Source: CAD feature listing. Evaluate the final solid. Frame: model axes, mm. Face numbers are marked on the shaded views. Give positions to 0.01 mm unless a question says otherwise; leave off trailing zeros. Write each loop counter-clockwise with the first axis right and the second up, starting at its lowest first coordinate (ties: lowest second). Pieces come first, ordered by that corner, then holes. Notation, with made-up numbers: (56.5, 31.5) -> (80.5, 31.5) arc R31 ccw to (80.5, 62.5) -> close; hole circle Ø7 at (82.25, -8). An arc over 180 degrees is marked (long way). Write item = value, one per line.
from build123d import *

# Parameters (mm, degrees)
BOSS_EXTRUDE1_DEPTH     = 432.4604
CUT_EXTRUDE1_DEPTH      = 18.43075
CUT_EXTRUDE1_DEPTH_BACK = 18.43075


with BuildPart() as part:
    # Sketch1 → Boss-Extrude1 (new body)
    with BuildSketch(Plane.XY):
        Polygon((-28.7655, -12.98575), (28.7655, -12.98575), (33.655, 17.43075), (38.1, 17.43075), (38.1, -17.43075), (-38.1, -17.43075), (-38.1, 17.43075), (-33.655, 17.43075), align=None)
    extrude(amount=BOSS_EXTRUDE1_DEPTH)

    # Sketch2 → Cut-Extrude1 (cut, two sides)
    with BuildSketch(Plane(origin=(0, 0, 0), x_dir=(1, 0, 0), z_dir=(0, 1, 0))) as cut_extrude1_sk:
        Polygon((-38.1, 0), (38.1, -129.9972), (38.1, 0), align=None)
        Polygon((-38.1, -432.4604), (38.1, -302.4632), (38.1, -432.4604), align=None)
    extrude(amount=CUT_EXTRUDE1_DEPTH, mode=Mode.SUBTRACT)
    extrude(cut_extrude1_sk.sketch, amount=-CUT_EXTRUDE1_DEPTH_BACK, mode=Mode.SUBTRACT)


solid = part.part
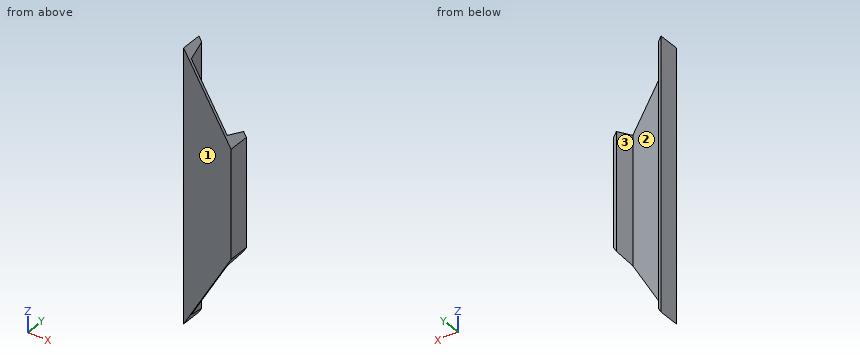
(1) First-contact query: pin 1 (6 mm diameter, centred on x = -21.5, z = 380, fed in from +Y); pin 2 (5 mm diameter, centred on y = 6, z = 65, fed in from +X). Flat tips, straight axial feed; report the tip coordinate or a pass-through.
Values follow:
pin_1 = -12.99
pin_2 = -31.42
(2) Section query B-B (z = 229.5). Return loops of the section in (x, y) (1 decimal), plus the area to 3 significant figures.
Values follow:
outline = (-38.1, -17.4) -> (38.1, -17.4) -> (38.1, 17.4) -> (33.7, 17.4) -> (28.8, -13) -> (-28.8, -13) -> (-33.7, 17.4) -> (-38.1, 17.4) -> close
area = 758 mm2
(3) Section query D-D (z = 382). Return loops of the section in (x, y) (1 decimal), plus the area to 3 significant figures.
Values follow:
outline = (-38.1, -17.4) -> (-8.5, -17.4) -> (-8.5, -13) -> (-28.8, -13) -> (-33.7, 17.4) -> (-38.1, 17.4) -> close
area = 341 mm2
(4) Section query A-A (y = 0). Return loops of the section in (x, z), plus the area to 3 significant figures.
Values follow:
outline = (-38.1, 0) -> (-30.85, 12.36) -> (-30.85, 420.1) -> (-38.1, 432.46) -> close; (30.85, 117.63) -> (38.1, 130) -> (38.1, 302.46) -> (30.85, 314.83) -> close
area = 4,380 mm2
(5) Section query C-C (x = 23.5). Return loops of the section in (y, z), plus the area to 3 significant figures.
Values follow:
outline = (-17.43, 105.09) -> (-12.99, 105.09) -> (-12.99, 327.37) -> (-17.43, 327.37) -> close
area = 988 mm2
(6) Pull-direction query (X, two-part tool) for the marked faces 1, 2 and 3; classes: pulls with the +X half, pulls with the -X half, needs draft (parallel to the pull), parting line crosses it, or undercut.
Values follow:
face_1 = needs draft
face_2 = undercut
face_3 = undercut
(7) Material intervals for line 1 (Y direction, x = -19, z = 394.5); line 2 (X direction, y = 14, z = 189); line 3 (X direction, y = 15, z = 224), sorted ascending.
Values follow:
line_1 = -17.43 to -12.99
line_2 = -38.1 to -33.1, 33.1 to 38.1
line_3 = -38.1 to -33.26, 33.26 to 38.1
